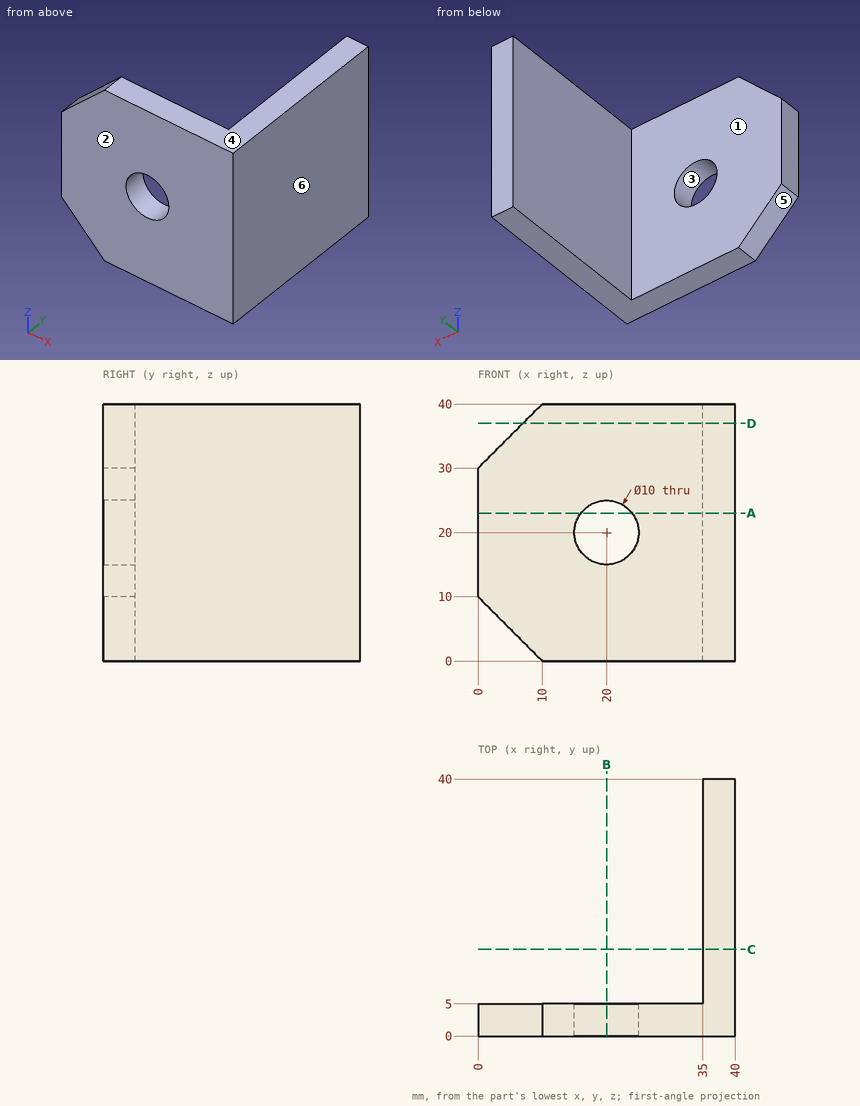
Can you work these out from the drawing? Everything is in mm from the part's minimum corner. A direction names the side the tool comes from. Round coordinates to 2 decimals unless told otherwise and drop trailing zeros. Loops run counter-clockwise (first coordinate to the right, second up) from the corner with the lowest first, then second, coordinate; pieces in that order, holes last. Notation, with made-up numbers: (-32.5, -23.5) -> (0.5, -23.5) arc R21 ccw to (0.5, -12.5) -> close; hole circle Ø10 at (-14, -16.5). An arc over 180 degrees is marked (long way). Answer in a Markdown table with one row per item.
Item 1: Will these pins go through, and if not, where does the flat tip stop? P1, Ø1.5, axis at y = 34.5, z = 24.5, coming from the -X side; P2, Ø6, axis at x = 25, z = 13, coming from the +Y side.
Answer block:
| item | result |
|---|---|
| P1 | x = 35 |
| P2 | y = 5 |
Item 2: Suppose I cut it at D-D, the plane z = 37. List the corners of the cut face in (x, y) for me, plus the area to 3 significant figures.
Answer block:
| item | result |
|---|---|
| outline | (7, 0) -> (40, 0) -> (40, 40) -> (35, 40) -> (35, 5) -> (7, 5) -> close |
| area | 340 mm² |
Item 3: Suppose I cut it at B-B, the plane x = 20. List the corners of the cut face in (y, z) for me.
Answer block:
| item | result |
|---|---|
| outline | (0, 0) -> (5, 0) -> (5, 15) -> (0, 15) -> close; (0, 25) -> (5, 25) -> (5, 40) -> (0, 40) -> close |
Item 4: Suppose I cut it at C-C, the plane y = 13.5. List the corners of the cut face in (x, z) for me, plus the area to 3 significant figures.
Answer block:
| item | result |
|---|---|
| outline | (35, 0) -> (40, 0) -> (40, 40) -> (35, 40) -> close |
| area | 200 mm² |
Item 5: On a 3-axis mill with a long thin cutter (end or side, diameter ignored), from which of +Z, -Z, +X, -X, +Y, -Y can I reach the whole of each face in a straight line? I mean the marked faces 1 and 2. Say none if no direction works.
Answer block:
| item | result |
|---|---|
| face 1 | +Z, -Z, -X, +Y |
| face 2 | +Z, -Z, +X, -X, -Y |
Item 6: Suppose I cut it at A-A, the plane z = 23. List the corners of the cut face in (x, y) for me, plus the area to 3 significant figures.
Answer block:
| item | result |
|---|---|
| outline | (0, 0) -> (16, 0) -> (16, 5) -> (0, 5) -> close; (24, 0) -> (40, 0) -> (40, 40) -> (35, 40) -> (35, 5) -> (24, 5) -> close |
| area | 335 mm² |
Item 7: If I drill on probe 1 along X at (y, z) = (1.45, 20); probe 2 along X at (y, z) = (23.5, 4); probe 3 along Y at (x, z) = (22.5, 33), over which ranges is the centre line in solid material (lowest first)?
Answer block:
| item | result |
|---|---|
| probe 1 | 0 to 15, 25 to 40 |
| probe 2 | 35 to 40 |
| probe 3 | 0 to 5 |
Item 8: We'd pull the mould along X, two halves only. Please class the marked faces 3, 4, 5 and 6: released by +X, released by -X, zero draft, split by the parting line, or undercut.
Answer block:
| item | result |
|---|---|
| face 3 | undercut |
| face 4 | zero draft |
| face 5 | released by -X |
| face 6 | released by +X |
